Input: dimensioned drawing with shaded views. Units: mm. Origin: part minimum x, y, z. A direction names the side the tool comes from. Round coordinates to 2 decimals unless told otherwise and drop trailing zeros. Write each loop counter-clockwise with the first axis right and the second up, starting at its lowest first coordinate (ties: lowest second). Pieces come first, ordered by that corner, then holes. Notation, with made-up numbers: (1, 43) -> (43, 43) arc R27 ccw to (43, 61) -> close; hole circle Ø7 at (45.25, 21.5). An arc over 180 degrees is marked (long way). One line per item, written item: value. Start each with the question number.
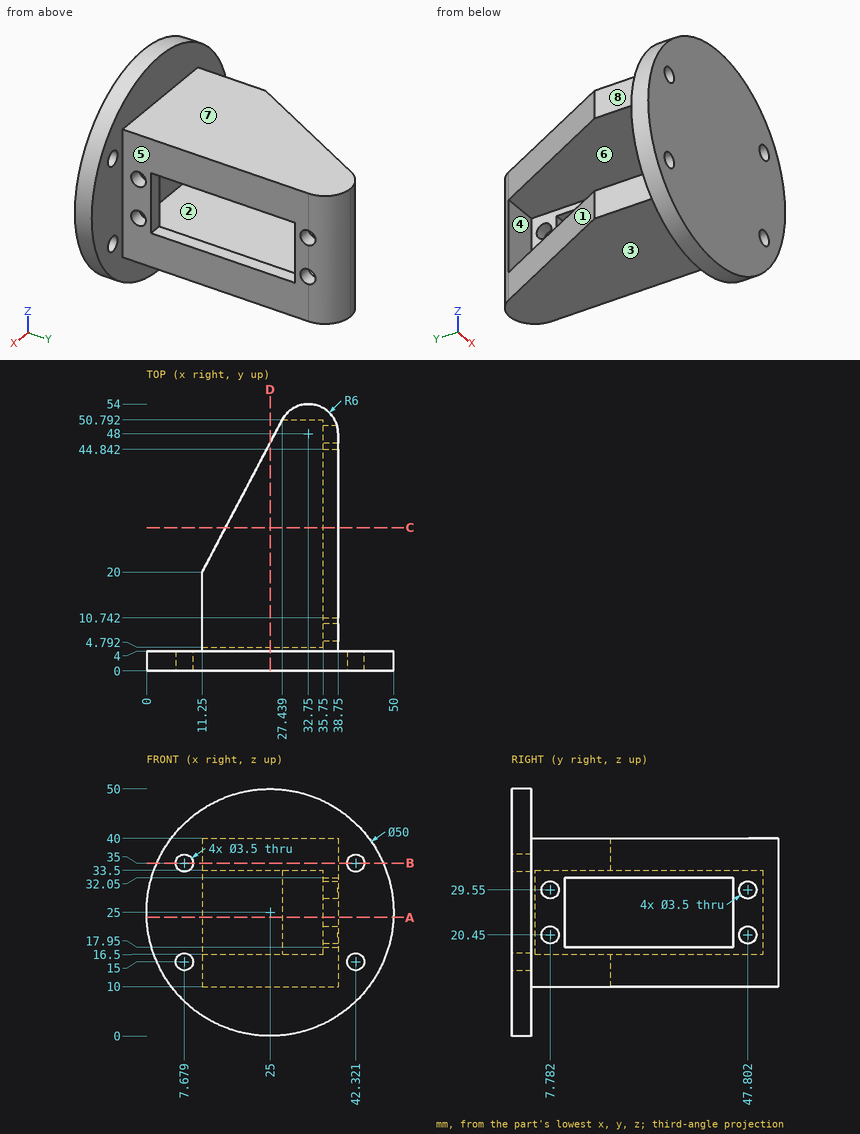
(1) Pull-direction query (Z, two-part tool) for the marked faces 1, 2, 3 and 4; classes: pulls with the +Z half, pulls with the -Z half, needs draft (parallel to the pull), parting line crosses it, or undercut.
(2) Line query: probe 1 along X at (y, z) = (1, 35); probe 2 along Z at (x, y) = (32.5, 50); probe 3 along Z at (x, y) = (38.5, 33.5). Output: solid intervals per line, ascending.
(3) Section query D-D (x = 25). Output: boundary loops of the cut face in (y, z).
(4) Section query B-B (z = 35). Output: boundary loops of the cut face in (x, y).
(5) Section query A-A (z = 24). Output: boundary loops of the cut face in (x, y), and give its area (3 significant figures).
(6) Pin query (flat end, axial travel): pin 1 (14 mm diameter, centred on x = 28, y = 34, fed in from -Z); pin 2 (2 mm diameter, centred on y = 14.5, z = 39.5, fed in from +X); pin 3 (3 mm diameter, centred on y = 47.8, z = 29.55, fed in from +X); pin 4 (10 mm diameter, centred on y = 45, z = 13, fed in from -X) (1 decimal). Return the tip coordinate at first contact, or that it passes through.
(7) Set-up query: the marked faces 5, 6, 7 and 8. Return all of +Z, -Z, +X, -X, +Y, -Y with unobstructed straight access to the full face (end or side cutting, diameter ignored); none if empty.
(8) Section query C-C (y = 29). Output: boundary loops of the cut face in (x, z), and give its area (3 significant figures).
Results list:
1. face 1: needs draft
1. face 2: undercut
1. face 3: pulls with the -Z half
1. face 4: undercut
2. probe 1: x = 2.09 to 5.93, 9.43 to 40.57, 44.07 to 47.91
2. probe 2: z = 10 to 16.5, 33.5 to 40
2. probe 3: z = 10 to 17.95, 32.05 to 40
3. outline: (0, 0) -> (4, 0) -> (4, 10) -> (46.15, 10) -> (46.15, 16.5) -> (4.79, 16.5) -> (4.79, 33.5) -> (46.15, 33.5) -> (46.15, 40) -> (4, 40) -> (4, 50) -> (0, 50) -> close
4. outline: (2.09, 0) -> (5.93, 0) -> (5.93, 4) -> (2.09, 4) -> close; (9.43, 0) -> (40.57, 0) -> (40.57, 4) -> (38.75, 4) -> (38.75, 48) arc R6 ccw to (27.44, 50.79) -> (11.25, 20) -> (11.25, 4) -> (9.43, 4) -> close; (44.07, 0) -> (47.91, 0) -> (47.91, 4) -> (44.07, 4) -> close
5. outline: (0.02, 0) -> (49.98, 0) -> (49.98, 4) -> (38.75, 4) -> (38.75, 10.74) -> (35.75, 10.74) -> (35.75, 4.79) -> (11.25, 4.79) -> (11.25, 4) -> (0.02, 4) -> close; (27.44, 50.79) -> (35.75, 50.79) -> (35.75, 44.84) -> (38.75, 44.84) -> (38.75, 48) arc R6 ccw to start
5. area: 281 mm^2
6. pin 1: stops at z = 10
6. pin 2: stops at x = 38.75
6. pin 3: passes through
6. pin 4: stops at x = 21.8
7. face 5: +Z, -Z, +X, +Y
7. face 6: -X
7. face 7: +Z, +X, -X, +Y
7. face 8: +Z, -Z, -X, +Y
8. outline: (15.98, 10) -> (38.75, 10) -> (38.75, 17.95) -> (35.75, 17.95) -> (35.75, 16.5) -> (15.98, 16.5) -> close; (15.98, 33.5) -> (35.75, 33.5) -> (35.75, 32.05) -> (38.75, 32.05) -> (38.75, 40) -> (15.98, 40) -> close
8. area: 305 mm^2
